```python
from build123d import *

# Parameters (mm, degrees)
CROQUIS1_W              = 300
CROQUIS1_H              = 200
SALIENTE_EXTRUIR1_DEPTH = 5
CROQUIS4_W              = 20
CROQUIS4_H              = 20
CORTAR_EXTRUIR4_DEPTH   = 10
CROQUIS5_W              = 150
CROQUIS5_H              = 120
CORTAR_EXTRUIR6_DEPTH   = 10


with BuildPart() as part:
    # Croquis1 → Saliente-Extruir1 (new body)
    with BuildSketch(Plane.XY):
        with Locations((-144.934554974, -91.263089005)):
            Rectangle(CROQUIS1_W, CROQUIS1_H)
    extrude(amount=SALIENTE_EXTRUIR1_DEPTH)

    # Croquis4 → Cortar-Extruir4 (cut)
    with BuildSketch(Plane.XY.offset(5)):
        with Locations((-284.934554974, -1.263089005)):
            Rectangle(CROQUIS4_W, CROQUIS4_H)
        with Locations((-4.934554974, -1.263089005)):
            Rectangle(CROQUIS4_W, CROQUIS4_H)
        with Locations((-284.934554974, -181.263089005)):
            Rectangle(CROQUIS4_W, CROQUIS4_H)
        with Locations((-4.934554974, -181.263089005)):
            Rectangle(CROQUIS4_W, CROQUIS4_H)
    extrude(amount=-CORTAR_EXTRUIR4_DEPTH, mode=Mode.SUBTRACT)

    # Croquis5 → Cortar-Extruir6 (cut)
    with BuildSketch(Plane.XY.offset(5)):
        with Locations((-144.934554974, -91.263089005)):
            Rectangle(CROQUIS5_W, CROQUIS5_H)
    extrude(amount=-CORTAR_EXTRUIR6_DEPTH, mode=Mode.SUBTRACT)


solid = part.part
```
Design review of the part built by this model. Coordinates are the model's own, in mm. Coordinates: 2 decimals unless noted, no trailing zeros. Order: outer loops, then holes, each group sorted by start corner. A loop starts at its lowest first (then second) coordinate and runs counter-clockwise, first axis right, second up.
1) Take a section at C-C, the plane y = -112. Give the boundary of the cut face in (x, z), and give its area (3 significant figures).
2) Clearance check with flat-ended pins moving along their axes: pin 1 (2.5 mm diameter, centred on y = -183, z = 1.5, fed in from -X); pin 2 (1.5 mm diameter, centred on x = -9.5, z = 1.5, fed in from -Y); pin 3 (1.5 mm diameter, centred on x = -280, z = 2.5, fed in from +Y). State where each tip first meets the part, or that it passes through.
3) Take a section at D-D, the plane y = -178. Give the boundary of the cut face in (x, z), and give its area (3 significant figures).
4) Take a section at B-B, the plane z = 1.2. Give the boundary of the cut face in (x, y).
5) Wall thickness on line 1 along X through (y, z) = (-102.5, 1.4); line 2 along Y through (x, z) = (-86, 2.55); line 3 along X through (y, z) = (-8.5, 4): over which ranges is each line inside the solid? List them lowest first.
6) Take a section at A-A, the plane x = -183. Give the boundary of the cut face in (y, z).
Returned:
1. outline: (-294.93, 0) - (-219.93, 0) - (-219.93, 5) - (-294.93, 5) - close; (-69.93, 0) - (5.07, 0) - (5.07, 5) - (-69.93, 5) - close
1. area: 750 mm2
2. pin 1: stops at x = -274.93
2. pin 2: stops at y = -171.26
2. pin 3: stops at y = -11.26
3. outline: (-274.93, 0) - (-14.93, 0) - (-14.93, 5) - (-274.93, 5) - close
3. area: 1,300 mm2
4. outline: (-294.93, -171.26) - (-274.93, -171.26) - (-274.93, -191.26) - (-14.93, -191.26) - (-14.93, -171.26) - (5.07, -171.26) - (5.07, -11.26) - (-14.93, -11.26) - (-14.93, 8.74) - (-274.93, 8.74) - (-274.93, -11.26) - (-294.93, -11.26) - close; hole (-219.93, -151.26) - (-69.93, -151.26) - (-69.93, -31.26) - (-219.93, -31.26) - close
5. line 1: x = -294.93 to -219.93, -69.93 to 5.07
5. line 2: y = -191.26 to -151.26, -31.26 to 8.74
5. line 3: x = -274.93 to -14.93
6. outline: (-191.26, 0) - (-151.26, 0) - (-151.26, 5) - (-191.26, 5) - close; (-31.26, 0) - (8.74, 0) - (8.74, 5) - (-31.26, 5) - close
